Solid Edge part; units mm, degrees
sketch "Sketch1" plane through (0, 0, 0) normal (1, 0, 0) x (0, 1, 0)
  line L0 (0, 0) -> (-30, 0)
  line L1 (-30, 0) -> (-30, -6.54)
  line L2 (-30, -6.54) -> (-50, -6.54)
  line L3 (-50, -6.54) -> (-50, -17.04)
  line L4 (-50, -17.04) -> (0, -17.04)
  line L5 (0, -17.04) -> (0, 0)
  dimension "D1" = 50
  dimension "D2" = 30
extrude "Protrusion1" add sketch "Sketch1" against normal blind 17
sketch "Sketch2" plane through (0, -25, -8.52) normal (1, 0, 0) x (0, 1, 0)
  spline S0 degree 3 poles (-71.3219, -134.81) (-69.7161, -64.7704) (-45.9422, -22.6838) (0, -8.52) knots 0 0 0 0 1 1 1 1
  line L0 (-25, 1.98) -> (0, -8.52)
  spline S1 degree 3 poles (-91.8715, -134.81) (-81.8395, -60.4295) (-62.3452, -13.2062) (-25, 1.98) knots 0 0 0 0 1 1 1 1
  line L1 (-91.8715, -134.81) -> (-71.3219, -134.81)
extrude "Extrusionsausprägung_2" add sketch "Sketch2" against normal blind 17
sketch "Sketch3" plane through (-8.5, -106.5967, -143.33) normal (0, 0, -1) x (0, 1, 0)
  circle A0 centre (0, 0) radius 3.2
extrude "Extrusionsausschnitt_1" cut sketch "Sketch3" against normal blind 9.5
mirror "Mirror1" about plane through (0, 0, 0) normal (0, -1, 0) of "Protrusion1", "Extrusionsausprägung_2", "Extrusionsausschnitt_1"
sketch "Sketch4" plane through (-8.5, -40, -6.54) normal (0, 0, 1) x (0, 1, 0)
  circle A0 centre (0, 1.5) radius 3.2
extrude "Extrusionsausschnitt_2" cut sketch "Sketch4" against normal blind 9.5
mirror "Mirror2" about plane through (0, 0, 0) normal (0, -1, 0) of "Extrusionsausschnitt_2"
properties part number "61" material "Polyacticacid"
Part model, mm, in its own coordinate system. A direction names the side the tool comes from. Give positions to 0.01 mm unless a question says otherwise; leave off trailing zeros. Write each loop counter-clockwise with the first axis right and the second up, starting at its lowest first coordinate (ties: lowest second). Pieces come first, ordered by that corner, then holes. Notation, with made-up numbers: M 37,29.5 L 74,29.5 A30 cw 74,65.5 Z; hole C -23.75,21.25 d1. An arc over 180 degrees is marked long. Use CSV: the item, a comma, the result in double quotes.
Item 1: Pull direction Y, two halves, no side cores. Call faces 5 (the face through (-8, 0, -17.04)), 6 (the face through (-8, -30, -3)), 7 (the face through (-9.461, 103.544, -138.646)), 8 (the face through (-6, 40, -6.54)): +Y half, -Y half, draft (parallel to the pull), parting line (faces both ways), or undercut.
Taken from the geometry:
face 5,"undercut"
face 6,"-Y half"
face 7,"undercut"
face 8,"draft"
Item 2: Which spindle directions (+Z, -Z, +X, -X, +Y, -Y) get a long thin tool onto all of the face, cutting with end or side? Do faces 1 (the face through (-9, 107, -133.83)), 2 (the face through (-6, -40, -6.54)), 3 (the face through (-7.84, 42.36, -11.22)), 4 (the face through (-8, 30, -3)). Say none if no direction does.
Taken from the geometry:
face 1,"-Z"
face 2,"+Z, +X, -X, -Y"
face 3,"+Z"
face 4,"+Z, +X, -X, +Y"
Item 3: Drill centre lines: probe 1 along X at (y, z) = (40, -10.25); probe 2 along Y at (x, z) = (-10, -12.5); probe 3 along Z at (x, y) = (-11, -12). Where is each one in solid material? Low to high.
Taken from the geometry:
probe 1,"x = -17 to -13.2, -6.8 to 0"
probe 2,"y = -61.37 to -43.2, -36.8 to 36.8, 43.2 to 61.37"
probe 3,"z = -17.04 to 0"
Item 4: Pin check, flat tips, straight feed: P1, Ø8.5, axis at x = -10, y = 40, coming from the +Z side; P2, Ø1, axis at x = -6.5, z = -53.5, coming from the +Y side; P3, Ø1, axis at x = -10.5, y = 54, coming from the +Z side. Stop position of each tip, or through.
Taken from the geometry:
P1,"stops at z = -6.54"
P2,"stops at y = 94.26"
P3,"stops at z = -8.08"
Item 5: Slice it at A-A on y = 15. Write the cut outline in (x, z).
Taken from the geometry:
outline,"M -17,-17.04 L 0,-17.04 L 0,0 L -17,0 Z"
Item 6: Slice it at B-B on z = -12. State how many separate pieces and enclosed holes the cut face has, plus the area to 3 significant figures.
Taken from the geometry:
separate pieces,"1"
enclosed holes,"2"
area,"2,000 mm²"
